Can you work these out from the model? Positions are in its coordinate system, mm. A direction names the side the tool comes from. Give positions to 0.01 mm unless a question says otherwise; leave off trailing zeros. Order: outer loops, then holes, each group sorted by start corner. A loop starts at its lowest first (then second) coordinate and runs counter-clockwise, first axis right, second up. Notation, with made-up numbers: M 24,-4 L 31,-4 A23 cw 31,20 Z; hole C 44.5,-27 d11. An arc over 180 degrees is marked long. Write each question's results on one line, items separated by ' | '.
from build123d import *

# Parameters (mm, degrees)
SKETCH1_R           = 2.5
SKETCH1_R_2         = 1.5
SKETCH1_R_3         = 3.5
BOSS_EXTRUDE1_DEPTH = 6.4
SKETCH2_R           = 3
CUT_EXTRUDE1_DEPTH  = 3
FILLET1_R           = 20
CHAMFER1_SIZE       = 5


with BuildPart() as part:
    # Sketch1 → Boss-Extrude1 (new body)
    with BuildSketch(Plane.XY):
        with BuildLine():
            Line((250, 19.05), (16.189425561, 19.05))
            ThreePointArc((16.189425561, 19.05), (-25, 0), (16.189425561, -19.05))
            Line((16.189425561, -19.05), (250, -19.05))
            Line((250, -19.05), (250, 19.05))
        make_face()
        with Locations((230, 0)):
            Circle(SKETCH1_R, mode=Mode.SUBTRACT)
        with Locations((210, 0)):
            Circle(SKETCH1_R, mode=Mode.SUBTRACT)
        with Locations((0, 12.7)):
            Circle(SKETCH1_R_2, mode=Mode.SUBTRACT)
        with Locations((12.7, 0)):
            Circle(SKETCH1_R_2, mode=Mode.SUBTRACT)
        with Locations((0, -12.7)):
            Circle(SKETCH1_R_2, mode=Mode.SUBTRACT)
        with Locations((-12.7, 0)):
            Circle(SKETCH1_R_2, mode=Mode.SUBTRACT)
        Circle(SKETCH1_R_3, mode=Mode.SUBTRACT)
    extrude(amount=BOSS_EXTRUDE1_DEPTH)

    # Sketch2 → Cut-Extrude1 (cut)
    with BuildSketch(Plane.XY.offset(6.4)):
        with Locations((0, 12.7)):
            Circle(SKETCH2_R)
        with Locations((12.7, 0)):
            Circle(SKETCH2_R)
        with Locations((0, -12.7)):
            Circle(SKETCH2_R)
        with Locations((-12.7, 0)):
            Circle(SKETCH2_R)
    extrude(amount=-CUT_EXTRUDE1_DEPTH, mode=Mode.SUBTRACT)

    # Fillet1
    fillet1_edges = [part.edges().sort_by_distance(p)[0] for p in [
        (16.189425561, -19.05, 3.2),
        (16.189425561, 19.05, 3.2),
    ]]
    fillet(fillet1_edges, radius=FILLET1_R)

    # Chamfer1
    chamfer1_edges = [part.edges().sort_by_distance(p)[0] for p in [
        (250, -19.05, 3.2),
        (250, 19.05, 3.2),
    ]]
    chamfer(chamfer1_edges, length=CHAMFER1_SIZE)


solid = part.part
(1) Imagine slicing it at A-A, the plane x = 90.5. Write out the boundary of the cut face in (y, z), plus the area to 3 significant figures.
Data:
outline: M -19.05,0 L 19.05,0 L 19.05,6.4 L -19.05,6.4 Z | area: 244 mm2
(2) We'd pull the mould along X, two halves only. Please class faces 4 (the face through (-11, -1, 3.4)), 5 (the face through (-24.99, 0.73, 3.16)), 6 (the face through (17.3, 19.7, 3.2)): +X half, -X half, draft (parallel to the pull), parting line (faces both ways), or undercut.
Data:
face 4: undercut | face 5: parting line | face 6: +X half
(3) Will these pins go through, and if not, where does the flat tip stop? P1, Ø1.8, axis at x = -12.5, y = -1.5, coming from the +Z side; P2, Ø2, axis at x = 170, z = 5.5, coming from the +Y side; P3, Ø3, axis at y = 4.5, z = 3.5, coming from the -X side.
Data:
P1: stops at z = 3.4 | P2: stops at y = 19.05 | P3: stops at x = -24.82
(4) For faces 1 (the face through (247.535, 16.515, 3.155)), 2 (the face through (11, -1, 3.4)), 3 (the face through (132, -19.05, 3)), which set-ups out of +Z, -Z, +X, -X, +Y, -Y let a thin tool reach every point of the face, with its end or its side?
Data:
face 1: +Z, -Z, +X, +Y | face 2: +Z | face 3: +Z, -Z, +X, -Y
(5) I need wall thicknesses on L1, parallel to Y at x = 0, z = 1.5; L2, parallel to Y at x = 230, z = 4.5; L3, parallel to Y at x = 13, z = 1.5. Which ranges of each line are inside material? Lowest first, please. Write a range as from..to.
Data:
L1: y = -25..-14.2, -11.2..-3.5, 3.5..11.2, 14.2..25 | L2: y = -19.05..-2.5, 2.5..19.05 | L3: y = -21.38..-1.47, 1.47..21.38
